Read the model definition and answer for the solid it produces. Units are mm, in the model's axes. Face numbers are marked on the shaded views. A direction names the side the tool comes from. Coordinates: 2 decimals unless noted, no trailing zeros. Order: outer loops, then holes, each group sorted by start corner. A loop starts at its lowest first (then second) coordinate and runs counter-clockwise, first axis right, second up. Notation, with made-up numbers: M 59.5,76.5 L 83.5,76.5 A17 ccw 83.5,102.5 Z; hole C -30.5,3.5 d10. An arc over 180 degrees is marked long. Write each question's results on one line, items separated by ' | '.
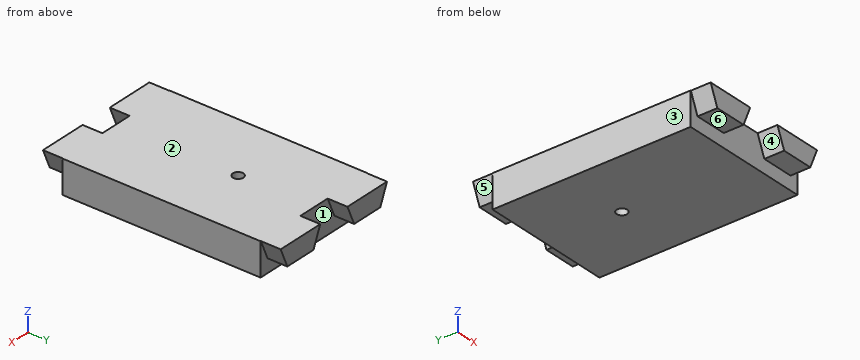
```python
from build123d import *

# Parameters (mm, degrees)
SKETCH_W     = 40
SKETCH_H     = 60
PAD_DEPTH    = 10
PAD001_DEPTH = 6
PAD002_DEPTH = 6
SKETCH003_R  = 1.6
POCKET_DEPTH = 10


with BuildPart() as part:
    # Sketch → Pad (new body)
    with BuildSketch(Plane.XY):
        with Locations((20, 30)):
            Rectangle(SKETCH_W, SKETCH_H)
    extrude(amount=PAD_DEPTH)

    # Sketch001 (on Face3 of Pad) → Pad001 (join)
    with BuildSketch(Plane.XZ):
        Polygon((0.1, 10), (14.9, 10), (12.4, 4.1), (2.6, 4.1), align=None)
        Polygon((25.1, 10), (39.9, 10), (37.4, 4.1), (27.6, 4.1), align=None)
    extrude(amount=PAD001_DEPTH)

    # Sketch002 (on Face1 of Pad001) → Pad002 (join)
    with BuildSketch(Plane(origin=(0, 60, 0), x_dir=(-1, 0, 0), z_dir=(0, 1, 0))):
        Polygon((-39.9, 10), (-25.1, 10), (-27.6, 4.1), (-37.4, 4.1), align=None)
        Polygon((-14.9, 10), (-0.1, 10), (-2.6, 4.1), (-12.4, 4.1), align=None)
    extrude(amount=PAD002_DEPTH)

    # Sketch003 (on Face4 of Pad002) → Pocket (cut)
    with BuildSketch(Plane.XY.offset(10)):
        with Locations((20, 37)):
            Circle(SKETCH003_R)
    extrude(amount=-POCKET_DEPTH, mode=Mode.SUBTRACT)


solid = part.part
```
(1) Given pin 1 (6.5 mm diameter, centred on x = 7.5, y = -4.5, fed in from -Z); pin 2 (3 mm diameter, centred on x = 22, z = 7, fed in from +Y), each flat-ended and moving along its own axis, determine where each tip first touches the part or whether it passes through.
Conclusion:
pin 1: z = 4.1 | pin 2: y = 60
(2) The part is cut by section C-C, the plane z = 1.75. Write down the section's boundary in (x, y).
Conclusion:
outline: M 0,0 L 40,0 L 40,60 L 0,60 Z; hole C 20,37 d3.2
(3) The part is cut by section A-A, the plane y = 37. Write down the section's boundary in (x, z), then the cut area to 3 significant figures.
Conclusion:
outline: M 0,0 L 18.4,0 L 18.4,10 L 0,10 Z; M 21.6,0 L 40,0 L 40,10 L 21.6,10 Z | area: 368 mm²
(4) For the marked faces 4, 5 and 6, determine the directions among +Z, -Z, +X, -X, +Y, -Y from which every point of the face is accessible in a straight line to the end or side of a thin tool.
Conclusion:
face 4: -Z, -Y | face 5: -Z, -X, +Y | face 6: -Z, +X, -X, -Y
(5) The mould has two halves that part along X. Classify the marked faces 1, 2 and 3: pulls with the +X half, pulls with the -X half, needs draft (parallel to the pull), parting line crosses it, or undercut.
Conclusion:
face 1: undercut | face 2: needs draft | face 3: pulls with the -X half
(6) Straight lines are drawn through the part: line 1 (Y direction, x = 20, z = 3.25); line 2 (Z direction, x = 8.5, y = 61.5); line 3 (Y direction, x = 17, z = 2). For each, find the intervals that lie inside material, in ascending order.
Conclusion:
line 1: 0 to 35.4, 38.6 to 60 | line 2: 4.1 to 10 | line 3: 0 to 60
(7) The part is cut by section B-B, the plane x = 20. Write down the section's boundary in (y, z), then the cut area to 3 significant figures.
Conclusion:
outline: M 0,0 L 35.4,0 L 35.4,10 L 0,10 Z; M 38.6,0 L 60,0 L 60,10 L 38.6,10 Z | area: 568 mm²
(8) The part is cut by section D-D, the plane x = 29. Write down the section's boundary in (y, z).
Conclusion:
outline: M -6,4.1 L 0,4.1 L 0,0 L 60,0 L 60,4.1 L 66,4.1 L 66,10 L -6,10 Z
